Autodesk Inventor part; units mm, degrees
ref_plane "YZ Plane" through (0, 0, 0) normal (1, 0, 0) x (0, 1, 0)
ref_plane "XZ Plane" through (0, 0, 0) normal (0, 1, 0) x (-1, 0, 0)
ref_plane "XY Plane" through (0, 0, 0) normal (0, 0, 1) x (1, 0, 0)
sketch "Sketch1" plane through (0, 0, 0) normal (1, 0, 0) x (0, 1, 0)
  line L0 (0, 0) -> (21.5526, 21.5526)
  line L1 (21.5526, 21.5526) -> (50.2894, -7.1842)
  line L2 (0, -101.8491) -> (0, 42.1347)
  line L3 (50.2894, -7.1842) -> (0, -57.4736)
  line L4 (0, 0) -> (0, -57.4736)
  line L5 (26.9408, 16.1645) -> (0, -10.7763) construction
  dimension "d0" = 40.64
  dimension "d1" = 45
  dimension "d5" = 7.62
  dimension "d6" = 38.1
extrude "Extrusion1" add sketch "Sketch1" along normal mid plane 40.64
sketch "Sketch2" plane through (-20.32, 21.5526, 21.5526) normal (0, 0.7071, 0.7071) x (1, 0, 0)
  line L0 (0, 0) -> (40.64, 0) construction
  line L1 (40.64, 0) -> (40.64, 40.64) construction
  line L2 (0, 0) -> (40.64, 40.64) construction
  line L3 (40.64, 40.64) -> (0, 40.64) construction
  line L4 (0, 40.64) -> (40.64, 0) construction
  line L5 (7.62, 7.62) -> (33.02, 7.62)
  line L6 (33.02, 7.62) -> (33.02, 33.02)
  line L7 (33.02, 33.02) -> (7.62, 33.02)
  line L8 (7.62, 33.02) -> (7.62, 7.62)
  line L9 (7.62, 7.62) -> (33.02, 33.02) construction
  line L10 (33.02, 7.62) -> (7.62, 33.02) construction
  point P0 (20.32, 0)
  point P1 (20.32, 20.32)
  dimension "d7" = 25.4
extrude "Extrusion2" cut sketch "Sketch2" against normal blind 38.1
sketch "Sketch3" plane through (0, 0, 0) normal (1, 0, 0) x (0, 1, 0)
  line L0 (21.5526, 21.5526) -> (0, 0)
  line L1 (0, 0) -> (0, -57.4736)
  line L2 (0, -57.4736) -> (50.2894, -7.1842)
  line L3 (17.9605, -28.7368) -> (0, -10.7763)
  line L4 (26.9408, 16.1645) -> (0, -10.7763)
  line L5 (0, 0) -> (0, -57.4736)
  line L6 (21.5526, 21.5526) -> (8.0019, 21.5526) construction
  line L7 (0, 0) -> (21.5526, 21.5526)
  line L8 (0, 0) -> (0, 46.9526)
  line L9 (50.2894, -7.1842) -> (0, -57.4736)
  line L10 (0, -57.4736) -> (0, -82.8736)
  line L11 (0, -137.4091) -> (0, 77.6947)
  line L12 (0, 46.9526) -> (-12.7, 46.9526)
  line L13 (-12.7, 46.9526) -> (-12.7, -82.8736)
  line L14 (-12.7, -82.8736) -> (0, -82.8736)
  point P0 (1.0999, -13.335)
  point P1 (0, -10.7763)
  dimension "d10" = 25.4
  dimension "d11" = 25.4
  dimension "d12" = 12.7
extrude "Extrusion3" add sketch "Sketch3" along normal mid plane 22.86
equation "\"d0\" = widthToSupportExtrusion"
equation "\"d1\" = attachementAngle"
equation "\"d6\" = insertDepth"
equation "\"d2\" = widthToSupportExtrusion"
equation "\"d7\" = extrusionSize"
equation "\"d8\" = insertDepth"
equation "\"d12\" = supportBaseDepth"
equation "\"d13\" = supportBaseWidth"
equation "\"attachementAngle\" = 45deg"
equation "\"extrusionSize\" = 25.4"
equation "\"wallThickness\" = 6.35"
equation "\"slipClearance\" = 1.27"
equation "\"insertForExtrusion\" = extrusionSize + 2 * slipClearance"
equation "\"widthToSupportExtrusion\" = insertForExtrusion + 2 * wallThickness"
equation "\"insertDepth\" = 38.1"
equation "\"supportBaseWidth\" = 22.86"
equation "\"supportBaseDepth\" = 12.7"
properties part number "45DegreeAttachementV02"
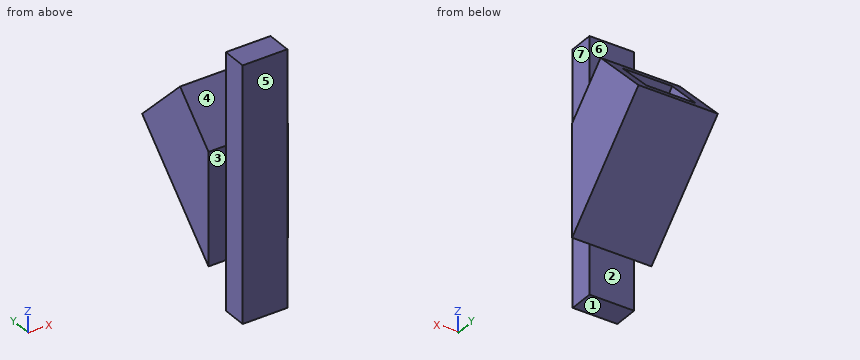
CAD build for the part. Positions are in the model's coordinates, mm. Face numbers are marked on the shaded views. A direction names the side the tool comes from. Coordinates: 2 decimals unless noted, no trailing zeros. Write each loop counter-clockwise with the first axis right and the second up, starting at its lowest first coordinate (ties: lowest second). Pieces come first, ordered by that corner, then holes.
(1) Flat gauge pins, fed straight in: pin 1 (5 mm diameter, centred on x = -13.5, y = 26, fed in from +Z); pin 2 (14 mm diameter, centred on y = -9, z = -44.5, fed in from -X); pin 3 (5 mm diameter, centred on x = 4, z = -46.5, fed in from +Y). Where does each tip first touch, or does it go through?
(2) Drill centre lines: probe 1 along X at (y, z) = (4, -10); probe 2 along Z at (x, y) = (11, 5.5); probe 3 along Y at (x, z) = (9.5, -61). Where is each one in solid material? Low to high.
(3) 3-axis set-ups, long thin cutter, end or side, ignore diameter. For the marked faces 1, 2, 3 and 4: which of +Z, -Z, +X, -X, +Y, -Y reach the whole face in a straight line?
(4) Two-plate mould, pull along Y, no slides. Class the marked faces 5, 6 and 7: +Y half, -Y half, draft (parallel to the pull), parting line (faces both ways), or undercut.
(5) Cut at A-A, the plane z = 9. List the corners of the cut face in (x, y).
(6) Cut at C-C, the plane y = 29. List the corners of the cut face in (x, z), and give its area (3 significant figures).
(7) Cut at D-D, the plane z = -75. List the corners of the cut face in (x, y), and give its area (3 significant figures).
Geometry says:
1. pin 1: stops at z = 19.61
1. pin 2: stops at x = -11.43
1. pin 3: stops at y = 13.47
2. probe 1: x = -20.32 to -12.7, 12.7 to 20.32
2. probe 2: z = -51.97 to -16.28, -5.28 to 5.5
2. probe 3: y = -12.7 to 0
3. face 1: -Z, +X, -X, +Y, -Y
3. face 2: -Z, +X, -X, +Y
3. face 3: +Z, -Z, -X, -Y
3. face 4: +Z, +X, -X
4. face 5: -Y half
4. face 6: undercut
4. face 7: draft
5. outline: (-20.32, 9) - (20.32, 9) - (20.32, 34.11) - (12.7, 34.11) - (12.7, 19.78) - (-12.7, 19.78) - (-12.7, 34.11) - (-20.32, 34.11) - close; (-11.43, -12.7) - (11.43, -12.7) - (11.43, 0) - (-11.43, 0) - close
6. outline: (-20.32, -28.47) - (20.32, -28.47) - (20.32, 14.11) - (12.7, 14.11) - (12.7, -17.7) - (-12.7, -17.7) - (-12.7, 14.11) - (-20.32, 14.11) - close
6. area: 923 mm2
7. outline: (-11.43, -12.7) - (11.43, -12.7) - (11.43, 0) - (-11.43, 0) - close
7. area: 290 mm2
